from build123d import *

# Parameters (mm, degrees)
ENLEV_MAT_EXTRU1_DEPTH = 1.3
ESQUISSE3_W            = 1.5
ESQUISSE3_H            = 8
CHANFREIN1_SIZE        = 0.3


with BuildPart() as part:
    # Esquisse1 → Base-Révolution (revolve)
    with BuildSketch(Plane(origin=(0, 0, 0), x_dir=(1, 0, 0), z_dir=(0, 1, 0)), mode=Mode.PRIVATE) as base_r_volution_sk:
        with BuildLine():
            Line((0, 0), (2.43, 0))
            Line((2.43, 0), (2.43, 1.45))
            ThreePointArc((2.43, 1.45), (2.415355339, 1.485355339), (2.38, 1.5))
            Line((2.38, 1.5), (0, 1.5))
            Line((0, 1.5), (0, 0))
        make_face()
    revolve(base_r_volution_sk.sketch.rotate(Axis((0, 0, 0), (0, 0, -1)), 180), axis=Axis((0, 0, 0), (0, 0, -1)))

    # Esquisse2 → enlev-mat-Extru1 (cut)
    with BuildSketch(Plane.XY.offset(-1.5)):
        Polygon((1.025891605, -0.592298794), (1.025891605, 0.592298794), (0, 1.184597588), (-1.025891605, 0.592298794), (-1.025891605, -0.592298794), (0, -1.184597588), align=None)
    extrude(amount=ENLEV_MAT_EXTRU1_DEPTH, mode=Mode.SUBTRACT)

    # Esquisse3 → Boss.-Révol.1 (revolve)
    with BuildSketch(Plane(origin=(0, 0, 0), x_dir=(1, 0, 0), z_dir=(0, 1, 0))):
        with Locations((0.75, -4)):
            Rectangle(ESQUISSE3_W, ESQUISSE3_H)
    revolve(axis=Axis((0, 0, 0), (0, 0, 1)))

    # Chanfrein1
    chanfrein1_edges = [part.edges().sort_by_distance(p)[0] for p in [
        (-1.5, 0, 8),
    ]]
    chamfer(chanfrein1_edges, length=CHANFREIN1_SIZE)


solid = part.part
For this review, take the finished solid that the model builds, in its own axes (mm). A direction names the side the tool comes from. Give positions to 0.01 mm unless a question says otherwise; leave off trailing zeros. Order: outer loops, then holes, each group sorted by start corner. A loop starts at its lowest first (then second) coordinate and runs counter-clockwise, first axis right, second up. Notation, with made-up numbers: M -8.5,-2.5 L -1.5,-2.5 A22 cw -1.5,9.5 Z; hole C 18.5,67.5 d11. An arc over 180 degrees is marked long. Answer in a Markdown table with one row per item. Add a question column.
(1) For faces 4 (the face through (0, -2, 0)), 5 (the face through (1, -1, -1.5)), 6 (the face through (0.51, -0.89, -0.86)), list the 3-axis set-ups (+Z, -Z, +X, -X, +Y, -Y) from which the entire face can be reached by the end or side of a thin tool; tool diameter is ignored.
(2) For pin 1 (2 mm diameter, centred on y = -0.5, z = 3, fed in from +X); pin 2 (2 mm diameter, centred on x = 1, y = 2, fed in from +Z); pin 3 (0.6 mm diameter, centred on x = 0, y = 0, fed in from -Z), all flat-tipped, find the tip position at first contact; note any pin that passes through.
(3) Consider section B-B on z = -0.5. State the section outline as (x, y) points.
(4) Consider section C-C on z = 4. State the section outline as (x, y) points.
(5) Consider section A-A on y = 0. State the section outline as (x, z) points, and give its area (3 significant figures).
(6) Wall thickness on probe 1 along Y at (x, z) = (0.05, 5.25); probe 2 along Z at (x, y) = (0.65, -1.4); probe 3 along Z at (x, y) = (0.1, 0.15): over which ranges is each line inside the solid? List them lowest first. Write a range as [from, to].
(7) Mouldability with a two-part tool opening along Y and no side actions: class faces 1 (the face through (-0.52, -0.884, -0.859)), 2 (the face through (0, 0, 8)), 3 (the face through (1.928, -1.479, -0.735)) as +Y half, -Y half, draft (parallel to the pull), parting line (faces both ways), or undercut.
Evaluation:
| question | item | result |
|---|---|---|
| 1 | face 4 | +Z |
| 1 | face 5 | -Z, +X, -X, +Y, -Y |
| 1 | face 6 | -Z |
| 2 | pin 1 | stops at x = 1.5 |
| 2 | pin 2 | stops at z = 7.96 |
| 2 | pin 3 | stops at z = -0.2 |
| 3 | outline | C 0,0 d4.86; hole M -1.03,-0.59 L 0,-1.18 L 1.03,-0.59 L 1.03,0.59 L 0,1.18 L -1.03,0.59 Z |
| 4 | outline | C 0,0 d3 |
| 5 | outline | M -2.43,-1.45 A0.05 ccw -2.38,-1.5 L -1.03,-1.5 L -1.03,-0.2 L 1.03,-0.2 L 1.03,-1.5 L 2.38,-1.5 A0.05 ccw 2.43,-1.45 L 2.43,0 L 1.5,0 L 1.5,7.7 L 1.2,8 L -1.2,8 L -1.5,7.7 L -1.5,0 L -2.43,0 Z |
| 5 | area | 28.5 mm^2 |
| 6 | probe 1 | y = [-1.5, 1.5] |
| 6 | probe 2 | z = [-1.5, 0] |
| 6 | probe 3 | z = [-0.2, 8] |
| 7 | face 1 | undercut |
| 7 | face 2 | draft |
| 7 | face 3 | parting line |
